For this review, take the finished solid that the model builds, in its own axes (mm). Face numbers are marked on the shaded views. A direction names the side the tool comes from. Give positions to 0.01 mm unless a question says otherwise; leave off trailing zeros. Loops run counter-clockwise (first coordinate to the right, second up) from the corner with the lowest first, then second, coordinate; pieces in that order, holes last.
```python
from build123d import *

# Parameters (mm, degrees)
F0_R     = 11.43
F1_DEPTH = 1.524
F2_R     = 4.0005
F3_DEPTH = 2.54
F4_R     = 1.778
F5_DEPTH = 25.4
F6_R     = 5.461
F6_R_2   = 4.0005
F7_DEPTH = 0.508


with BuildPart() as f1:
    # F0 (on Top) → F1 (new body)
    with BuildSketch(Plane.XY):
        Circle(F0_R)
    extrude(amount=F1_DEPTH)

    # F2 (on face) → F3 (join)
    with BuildSketch(Plane.XY.offset(1.524)):
        Circle(F2_R)
    extrude(amount=F3_DEPTH)

    # F4 (on face) → F5 (cut)
    with BuildSketch(Plane.XY.offset(4.064)):
        Circle(F4_R)
    extrude(amount=-F5_DEPTH, mode=Mode.SUBTRACT)

    # F6 (on face) → F7 (join)
    with BuildSketch(Plane.XY.offset(1.524)):
        Circle(F6_R)
        Circle(F6_R_2, mode=Mode.SUBTRACT)
    extrude(amount=F7_DEPTH)


solid = f1.part
```
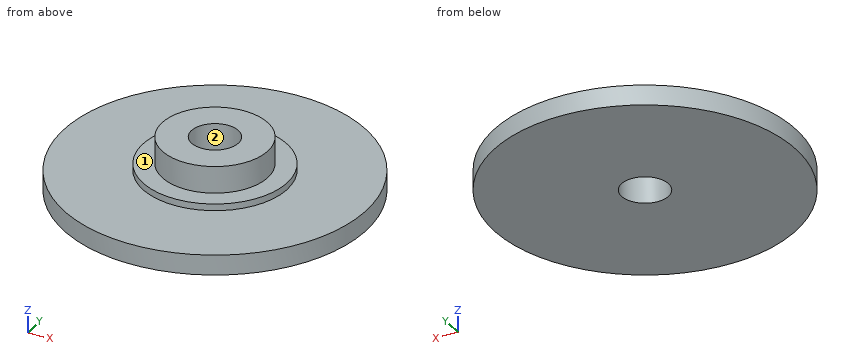
Q1. For probe 1 along Y at (x, z) = (0, 0.9); probe 2 along Y at (x, z) = (0, 2.65); probe 3 along Z at (x, y) = (-9.75, 4.25), list the stretches that pass through material, from the lowest coordinate up.
Answers:
probe 1: y = -11.43 to -1.78, 1.78 to 11.43
probe 2: y = -4 to -1.78, 1.78 to 4
probe 3: z = 0 to 1.52
Q2. Consider section D-D on y = 3.25. Give the boundary of the cut face in (x, z), plus the area to 3 significant figures.
Answers:
outline: (-10.96, 0) - (10.96, 0) - (10.96, 1.52) - (4.39, 1.52) - (4.39, 2.03) - (2.33, 2.03) - (2.33, 4.06) - (-2.33, 4.06) - (-2.33, 2.03) - (-4.39, 2.03) - (-4.39, 1.52) - (-10.96, 1.52) - close
area: 47.3 mm2
Q3. For pin 1 Ø2 at (x, y) = (0, 0) entering from -Z, flat-tipped, find the tip position at first contact; note if it passes through.
Answers:
pin 1: passes through
Q4. Machinability: for the marked faces 1 and 2, which of the approach directions +Z, -Z, +X, -X, +Y, -Y give a long, thin tool a straight path to every point of the face, cutting with its end or side? Answer none if there is none.
Answers:
face 1: +Z
face 2: +Z, -Z
Q5. Consider section A-A on y = 0. Give the boundary of the cut face in (x, z), plus the area to 3 significant figures.
Answers:
outline: (-11.43, 0) - (-1.78, 0) - (-1.78, 4.06) - (-4, 4.06) - (-4, 2.03) - (-5.46, 2.03) - (-5.46, 1.52) - (-11.43, 1.52) - close; (1.78, 0) - (11.43, 0) - (11.43, 1.52) - (5.46, 1.52) - (5.46, 2.03) - (4, 2.03) - (4, 4.06) - (1.78, 4.06) - close
area: 42.2 mm2
Q6. Consider section C-C on z = 0.5. Give the boundary of the cut face in (x, y), plus the area to 3 significant figures.
Answers:
outline: circle Ø22.86 at (0, 0); hole circle Ø3.56 at (0, 0)
area: 401 mm2
